```python
from build123d import *

# Parameters (mm, degrees)
SKETCH1_W                 = 50
SKETCH1_H                 = 40
BOSS_EXTRUDE1_DEPTH       = 40
CUT_EXTRUDE1_REACH        = 42
SKETCH2_W                 = 30
SKETCH2_H                 = 30
SKETCH3_R                 = 13
CUT_EXTRUDE2_DEPTH        = 6
SKETCH4_R                 = 13
CUT_EXTRUDE3_DEPTH        = 6
M3X0_5_TAPPED_HOLE1_D     = 2.5
M3X0_5_TAPPED_HOLE1_DEPTH = 6.5
M3X0_5_TAPPED_HOLE1_TIP   = 0.751075774
M3X0_5_TAPPED_HOLE2_D     = 2.5
M3X0_5_TAPPED_HOLE2_DEPTH = 6.5
M3X0_5_TAPPED_HOLE2_TIP   = 0.751075774
M3X0_5_TAPPED_HOLE3_D     = 2.5
M3X0_5_TAPPED_HOLE3_DEPTH = 4
M3X0_5_TAPPED_HOLE3_TIP   = 0.751075774
SKETCH13_R                = 4
CUT_EXTRUDE4_DEPTH        = 8
SKETCH15_W                = 4
SKETCH15_H                = 5
CUT_EXTRUDE5_DEPTH        = 6
SKETCH16_W                = 4
SKETCH16_H                = 5
CUT_EXTRUDE6_DEPTH        = 6
M3X0_5_TAPPED_HOLE4_D     = 2.5
M3X0_5_TAPPED_HOLE4_DEPTH = 6.5
M3X0_5_TAPPED_HOLE4_TIP   = 0.751075774
M3X0_5_TAPPED_HOLE5_D     = 2.5
M3X0_5_TAPPED_HOLE5_DEPTH = 6.5
M3X0_5_TAPPED_HOLE5_TIP   = 0.751075774


with BuildPart() as part:
    # Sketch1 → Boss-Extrude1 (new body)
    with BuildSketch(Plane(origin=(0, 0, 0), x_dir=(1, 0, 0), z_dir=(0, 1, 0))):
        Rectangle(SKETCH1_W, SKETCH1_H)
    extrude(amount=BOSS_EXTRUDE1_DEPTH)

    # Sketch2 → Cut-Extrude1 (cut, up to next)
    with BuildSketch(Plane(origin=(0, 40, 0), x_dir=(1, 0, 0), z_dir=(0, 1, 0)), mode=Mode.PRIVATE) as cut_extrude1_sk1:
        with Locations((0, -5)):
            Rectangle(SKETCH2_W, SKETCH2_H)
    cut_extrude1_tool1 = extrude(cut_extrude1_sk1.sketch, amount=-CUT_EXTRUDE1_REACH, mode=Mode.PRIVATE) & part.part
    add(cut_extrude1_tool1.solids().sort_by_distance((0, 40, 5))[0], mode=Mode.SUBTRACT)

    # Sketch3 → Cut-Extrude2 (cut)
    with BuildSketch(Plane.ZY.offset(25)):
        with Locations((5, 20)):
            Circle(SKETCH3_R)
    extrude(amount=-CUT_EXTRUDE2_DEPTH, mode=Mode.SUBTRACT)

    # Sketch4 → Cut-Extrude3 (cut)
    with BuildSketch(Plane(origin=(25, 0, 0), x_dir=(0, 0, -1), z_dir=(1, 0, 0))):
        with Locations((-5, 20)):
            Circle(SKETCH4_R)
    extrude(amount=-CUT_EXTRUDE3_DEPTH, mode=Mode.SUBTRACT)

    # M3x0.5 Tapped Hole1
    with Locations(Plane.ZY.offset(19)):
        with Locations((5, 30), (5, 10)):
            Hole(M3X0_5_TAPPED_HOLE1_D / 2, depth=M3X0_5_TAPPED_HOLE1_DEPTH)
            with Locations((0, 0, -(M3X0_5_TAPPED_HOLE1_DEPTH + M3X0_5_TAPPED_HOLE1_TIP / 2))):  # 118° drill point
                Cone(0, M3X0_5_TAPPED_HOLE1_D / 2, M3X0_5_TAPPED_HOLE1_TIP, mode=Mode.SUBTRACT)

    # M3x0.5 Tapped Hole2
    with Locations(Plane(origin=(19, 0, 0), x_dir=(0, 0, -1), z_dir=(1, 0, 0))):
        with Locations((-5, 30), (-5, 10)):
            Hole(M3X0_5_TAPPED_HOLE2_D / 2, depth=M3X0_5_TAPPED_HOLE2_DEPTH)
            with Locations((0, 0, -(M3X0_5_TAPPED_HOLE2_DEPTH + M3X0_5_TAPPED_HOLE2_TIP / 2))):  # 118° drill point
                Cone(0, M3X0_5_TAPPED_HOLE2_D / 2, M3X0_5_TAPPED_HOLE2_TIP, mode=Mode.SUBTRACT)

    # M3x0.5 Tapped Hole3
    with Locations(Plane.XY.offset(20)):
        with Locations((-20, 30), (-20, 10), (20, 10), (20, 30)):
            Hole(M3X0_5_TAPPED_HOLE3_D / 2, depth=M3X0_5_TAPPED_HOLE3_DEPTH)
            with Locations((0, 0, -(M3X0_5_TAPPED_HOLE3_DEPTH + M3X0_5_TAPPED_HOLE3_TIP / 2))):  # 118° drill point
                Cone(0, M3X0_5_TAPPED_HOLE3_D / 2, M3X0_5_TAPPED_HOLE3_TIP, mode=Mode.SUBTRACT)

    # Sketch13 → Cut-Extrude4 (cut)
    with BuildSketch(Plane.XY.offset(-10)):
        with Locations((0, 20)):
            Circle(SKETCH13_R)
    extrude(amount=-CUT_EXTRUDE4_DEPTH, mode=Mode.SUBTRACT)

    # Sketch15 → Cut-Extrude5 (cut)
    with BuildSketch(Plane(origin=(25, 0, 0), x_dir=(0, 0, -1), z_dir=(1, 0, 0))):
        with Locations((-18, 20)):
            Rectangle(SKETCH15_W, SKETCH15_H)
    extrude(amount=-CUT_EXTRUDE5_DEPTH, mode=Mode.SUBTRACT)

    # Sketch16 → Cut-Extrude6 (cut)
    with BuildSketch(Plane.ZY.offset(25)):
        with Locations((18, 20)):
            Rectangle(SKETCH16_W, SKETCH16_H)
    extrude(amount=-CUT_EXTRUDE6_DEPTH, mode=Mode.SUBTRACT)

    # M3x0.5 Tapped Hole4
    with Locations(Plane.ZY.offset(25)):
        with Locations((-7, 35), (-7, 5), (17, 5), (17, 35)):
            Hole(M3X0_5_TAPPED_HOLE4_D / 2, depth=M3X0_5_TAPPED_HOLE4_DEPTH)
            with Locations((0, 0, -(M3X0_5_TAPPED_HOLE4_DEPTH + M3X0_5_TAPPED_HOLE4_TIP / 2))):  # 118° drill point
                Cone(0, M3X0_5_TAPPED_HOLE4_D / 2, M3X0_5_TAPPED_HOLE4_TIP, mode=Mode.SUBTRACT)

    # M3x0.5 Tapped Hole5
    with Locations(Plane(origin=(25, 0, 0), x_dir=(0, 0, -1), z_dir=(1, 0, 0))):
        with Locations((-17, 35), (7, 35), (7, 5), (-17, 5)):
            Hole(M3X0_5_TAPPED_HOLE5_D / 2, depth=M3X0_5_TAPPED_HOLE5_DEPTH)
            with Locations((0, 0, -(M3X0_5_TAPPED_HOLE5_DEPTH + M3X0_5_TAPPED_HOLE5_TIP / 2))):  # 118° drill point
                Cone(0, M3X0_5_TAPPED_HOLE5_D / 2, M3X0_5_TAPPED_HOLE5_TIP, mode=Mode.SUBTRACT)


solid = part.part
```
Geometry check sheet. Reference: the model listing, model coordinates, mm. A direction names the side the tool comes from. Coordinates: 2 decimals unless noted, no trailing zeros. Order: outer loops, then holes, each group sorted by start corner. A loop starts at its lowest first (then second) coordinate and runs counter-clockwise, first axis right, second up.
Item 1: Section check D-D (x = 0). Enter the section's corners in (y, z), plus the area to 3 significant figures.
Item 2: Depth check by flat-ended pin: pin 1 (9 mm diameter, centred on y = 23.5, z = 7.5, fed in from +X); pin 2 (6 mm diameter, centred on y = 11, z = 0, fed in from +X); pin 3 (2 mm diameter, centred on x = 20, y = 30, fed in from +Z); pin 4 (7 mm diameter, centred on x = 0, y = 20, fed in from +Z). Enter the tip coordinate at first touch or a pass-through.
Item 3: Tool access check on faces 1 (the cylindrical face through (-16.97, 11.24, 5.16)), 2 (the cylindrical face through (-21.704, 33.891, 16.423)), 3 (the cylindrical face through (-21.155, 29.521, 17.972)), 4 (the flat face through (-22, 17.5, 19)). Record the directions out of +Z, -Z, +X, -X, +Y, -Y that give a thin tool (end or side, any length) a straight path to the whole face; none if there is none.
Item 4: Section check C-C (z = 5). Count the separate pieces of the cut face and the enclosed holes in it, plus the area to 3 significant figures.
Item 5: Scan lines: line 1 along X through (y, z) = (10, 19.15); line 2 along Y through (x, z) = (-20, -7); line 3 along Y through (x, z) = (17.95, 5). Record each from-to range of solid material in increasing order.
Item 6: Section check B-B (z = -15). Enter the section's corners in (x, y).
Item 7: Section check A-A (z = -9). Enter the section's corners in (x, y).
Item 8: Mould release check, pull along Y, two halves, no side actions. Record for faces 5 (the cylindrical face through (21.7, 33.78, 16.73)), 6 (the flat face through (25, 20, -9)), 7 (the conical face through (-17.88, 5.07, 17.21)), 8 (the flat face through (0, 40, -14)): released by +Y, released by -Y, zero draft, split by the parting line, or undercut.
Check sheet entries:
1. outline: (0, -20) - (40, -20) - (40, -10) - (24, -10) - (24, -18) - (16, -18) - (16, -10) - (0, -10) - close
1. area: 336 mm2
2. pin 1: stops at x = 19
2. pin 2: stops at x = 25
2. pin 3: stops at z = 15.85
2. pin 4: stops at z = -18
3. face 1: +X, -X
3. face 2: -X
3. face 3: +Z
3. face 4: +Z, -X
4. separate pieces: 6
4. enclosed holes: 0
4. area: 448 mm2
5. line 1: x = -25 to -21.25, -18.75 to -15, 15 to 18.75, 21.25 to 25
5. line 2: y = 0 to 3.75, 6.25 to 15, 25 to 33.75, 36.25 to 40
5. line 3: y = 0 to 8.75, 11.25 to 28.75, 31.25 to 40
6. outline: (-25, 0) - (25, 0) - (25, 40) - (-25, 40) - close; hole circle Ø8 at (0, 20)
7. outline: (-25, 0) - (-15, 0) - (-15, 40) - (-25, 40) - close; (15, 0) - (25, 0) - (25, 40) - (15, 40) - close
8. face 5: undercut
8. face 6: zero draft
8. face 7: undercut
8. face 8: released by +Y
